Autodesk Inventor part; units mm, degrees
ref_plane "YZ Plane" through (0, 0, 0) normal (1, 0, 0) x (0, 1, 0)
ref_plane "XZ Plane" through (0, 0, 0) normal (0, 1, 0) x (-1, 0, 0)
ref_plane "XY Plane" through (0, 0, 0) normal (0, 0, 1) x (1, 0, 0)
sketch "Sketch1" plane through (0, 0, 0) normal (0, 1, 0) x (-1, 0, 0)
  line L0 (58, 27) -> (-58, 27)
  line L1 (-58, 27) -> (-58, -27)
  line L2 (-58, -27) -> (58, -27)
  line L3 (58, -27) -> (58, 27)
  line L4 (58, 27) -> (-58, -27) construction
  line L5 (-58, 27) -> (58, -27) construction
  point P0 (0, 0)
  dimension "d0" = 116
  dimension "d1" = 54
extrude "Body" add sketch "Sketch1" along normal mid plane 10
sketch "Sketch2" plane through (0, 5, 0) normal (0, 1, 0) x (1, 0, 0)
  line L0 (-55.75, 18.75) -> (55.75, 18.75)
  line L1 (55.75, 18.75) -> (55.75, -18.75)
  line L2 (55.75, -18.75) -> (-55.75, -18.75)
  line L3 (-55.75, -18.75) -> (-55.75, 18.75)
  line L4 (-55.75, 18.75) -> (55.75, -18.75) construction
  line L5 (55.75, 18.75) -> (-55.75, -18.75) construction
  point P0 (0, 0)
  dimension "d4" = 111.5
  dimension "d5" = 37.5
extrude "Top Socket" cut sketch "Sketch2" against normal blind 2
sketch "Sketch3" plane through (0, 3, 0) normal (0, 1, 0) x (1, 0, 0)
  line L0 (-8, -9) -> (8, -9)
  line L1 (8, -9) -> (8, 9)
  line L2 (8, 9) -> (-8, 9)
  line L3 (-8, 9) -> (-8, -9)
  line L4 (-8, -9) -> (8, 9) construction
  line L5 (8, -9) -> (-8, 9) construction
  point P0 (0, 0)
  dimension "d29" = 18
  dimension "d30" = 16
extrude "Photoelectrode Bay" cut sketch "Sketch3" against normal blind 2
sketch "Sketch4" plane through (0, 3, 0) normal (0, 1, 0) x (1, 0, 0)
  circle A0 centre (14, 0) radius 1.45
  line L0 (-55.75, -18.75) -> (-55.75, 18.75)
  line L1 (-55.75, 0) -> (55.75, 0)
  line L2 (55.75, 18.75) -> (55.75, -18.75)
  line L3 (-55.75, -3) -> (55.75, -3)
  line L4 (8, 9) -> (8, -9)
  point P0 (0, 0)
  dimension "d11" = 2.9
  dimension "d20" = 3
  dimension "d97" = 6
revolve "Ref elec" cut sketch "Sketch4" angle 90 about axis through (-55.75, 3, 3) along (-1, 0, 0) contours L1 A0 | A0 L1
sketch "Sketch7" plane through (-58, 5, 27) normal (0, 0, 1) x (1, 0, 0)
  circle A0 centre (72, -5) radius 1.45
  circle A1 centre (72, -5) radius 1.45
  point P0 (58, -5)
  dimension "d21" = 2.9
extrude "Ref elec length" cut sketch "Sketch7" against normal up to surface (24 mm away)
sketch "Sketch8" plane through (-58, 5, 27) normal (0, 0, 1) x (1, 0, 0)
  line L0 (116, -10) -> (0, -10)
  line L1 (113.75, 0) -> (2.25, 0)
  line L2 (64.5, 0) -> (79.5, 0)
  line L3 (79.5, 0) -> (79.5, -10)
  line L4 (79.5, -10) -> (64.5, -10)
  line L5 (64.5, -10) -> (64.5, 0)
  line L6 (79.5, 0) -> (64.5, -10) construction
  line L7 (116, -10) -> (116, 0)
  point P0 (58, -5)
  point P1 (72, -5)
  point P2 (72, -10)
  dimension "d108" = 15
  dimension "d109" = 0
sketch "Sketch9" plane through (0, 1, 0) normal (0, 1, 0) x (1, 0, 0)
  line L0 (8, -9) -> (-8, -9)
  line L1 (8, -9) -> (-8, -9)
  line L2 (-8, -9) -> (8, -9)
  line L3 (8, -9) -> (8, -5.5)
  line L4 (8, -5.5) -> (-8, -5.5)
  line L5 (-8, -5.5) -> (-8, -9)
  dimension "d70" = 3.5
extrude "Photoelectrode Hole" cut sketch "Sketch9" against normal through all
sketch "Sketch12" plane through (0, 5, 0) normal (0, 1, 0) x (1, 0, 0)
  line L0 (58, 27) -> (-58, 27)
  circle A0 centre (-50.8, 25.4) radius 6
  line L1 (-58, -27) -> (-58, 27)
  line L2 (-58, 0) -> (58, 0)
  line L3 (58, 27) -> (58, -27)
  line L4 (-58, -27) -> (58, -27)
  line L5 (0, -27) -> (0, 27)
  circle A1 centre (50.8, 25.4) radius 6
  circle A2 centre (-50.8, -25.4) radius 6
  circle A3 centre (50.8, -25.4) radius 6
  line L6 (-50.8, 25.4) -> (50.8, 25.4)
  line L7 (-50.8, -25.4) -> (50.8, -25.4)
  circle A4 centre (0, 25.4) radius 6
  circle A5 centre (0, -25.4) radius 6
  point P0 (0, 0)
  dimension "d40" = 25.4
  dimension "d49" = 50.8
  dimension "d57" = 12
extrude "Screw clamp boss" add sketch "Sketch12" against normal up to surface (10 mm away) contours A1 L0 | L0 A1 | A4 L6 L5 L0 | L0 A4 | A5 L7 L5 | L5 L7 A5 | A4 L6 L5 | L5 L6 A4 | A3 L4 | L4 A3 | L5 L6 A4 L0 | L7 A5 L4 L5 | L5 L4 A5 L7 | A0 L0 | L0 A0 | A2 L4 | L4 A2 | L4 A5
sketch "Sketch15" plane through (0, 5, 0) normal (0, 1, 0) x (1, 0, 0)
  circle A0 centre (0, 25.4) radius 3.5
  arc A1 (5.7827, 27) -> (-5.7827, 27) centre (0, 25.4) ccw
  circle A2 centre (-50.8, 25.4) radius 3.5
  arc A3 (-45.0173, 27) -> (-56.5827, 27) centre (-50.8, 25.4) ccw
  line L0 (55.75, -18.75) -> (-55.75, -18.75)
  line L1 (0, -18.75) -> (0, 18.75)
  line L2 (-55.75, 18.75) -> (55.75, 18.75)
  line L3 (-58, 27) -> (-58, -27)
  line L4 (-58, 0) -> (58, 0)
  line L5 (58, -27) -> (58, 27)
  circle A4 centre (50.8, 25.4) radius 3.5
  circle A5 centre (0, -25.4) radius 3.5
  circle A6 centre (-50.8, -25.4) radius 3.5
  circle A7 centre (50.8, -25.4) radius 3.5
  point P0 (0, 0)
  dimension "d60" = 7
extrude "Screw Clamp Hole" cut sketch "Sketch15" against normal through all
sketch "Sketch18" plane through (-0.0162, 3, 0) normal (0, 1, 0) x (1, 0, 0)
  line L0 (-45, -15) -> (45, -15)
  line L1 (50, -10) -> (50, 10)
  line L2 (45, 15) -> (-45, 15)
  line L3 (-50, 10) -> (-50, -10)
  line L4 (-50, -15) -> (50, 15) construction
  line L5 (50, -15) -> (-50, 15) construction
  line L6 (-45, -15.5) -> (45, -15.5)
  line L7 (50.5, -10) -> (50.5, 10)
  line L8 (45, 15.5) -> (-45, 15.5)
  line L9 (-50.5, 10) -> (-50.5, -10)
  line L10 (-50.5, -15.5) -> (50.5, 15.5) construction
  line L11 (50.5, -15.5) -> (-50.5, 15.5) construction
  arc A0 (-50, -10) -> (-45, -15) centre (-45, -10) ccw
  arc A1 (45, -15) -> (50, -10) centre (45, -10) ccw
  arc A2 (50, 10) -> (45, 15) centre (45, 10) ccw
  arc A3 (-45, 15) -> (-50, 10) centre (-45, 10) ccw
  arc A4 (-50.5, -10) -> (-45, -15.5) centre (-45, -10) ccw
  arc A5 (45, -15.5) -> (50.5, -10) centre (45, -10) ccw
  arc A6 (50.5, 10) -> (45, 15.5) centre (45, 10) ccw
  arc A7 (-45, 15.5) -> (-50.5, 10) centre (-45, 10) ccw
  point P0 (0, 0)
  dimension "d83" = 100
  dimension "d84" = 30
  dimension "d85" = 0.5
  dimension "d86" = 0.5
  dimension "d87" = 5
  dimension "d88" = 5
  dimension "d89" = 5
  dimension "d90" = 5
  dimension "d91" = 5.5
  dimension "d92" = 5.5
  dimension "d93" = 5.5
  dimension "d94" = 5.5
extrude "Knife Edge" add sketch "Sketch18" along normal blind 1
extrude "Ref Electrode Outlet" add sketch "Sketch8" along normal blind 15
sketch "Sketch19" plane through (45.0173, -5, 27) normal (0, 0, 1) x (1, 0, 0)
  circle A0 centre (-31.0173, 5) radius 1.45
  circle A1 centre (-31.0173, 5) radius 1.45
  line L0 (0, 10) -> (-39.2345, 10)
  line L1 (-29.5673, 10) -> (-18.6963, 10)
  line L2 (-23.5173, 10) -> (0, 10)
  point P0 (-45.0173, 5)
extrude "Extrusion22" cut sketch "Sketch19" along normal blind 9.5
sketch "Sketch20" plane through (0, 5, 0) normal (0, 1, 0) x (1, 0, 0)
  circle A0 centre (14, -35.05) radius 1.45
  circle A1 centre (14, 0) radius 1.45
  line L0 (12.55, -36.5) -> (15.45, -36.5)
  point P0 (0, 0)
extrude "Extrusion23" cut sketch "Sketch20" against normal blind 5 contours A0
sketch "Sketch21" plane through (0, 5, 0) normal (0, 1, 0) x (1, 0, 0)
  circle A0 centre (14, -35.05) radius 4
  circle A1 centre (14, -35.05) radius 1.45
  line L0 (10, -39.05) -> (18, -39.05)
  line L1 (18, -39.05) -> (18, -31.05)
  line L2 (18, -31.05) -> (10, -31.05)
  line L3 (10, -31.05) -> (10, -39.05)
  line L4 (10, -39.05) -> (18, -31.05) construction
  line L5 (18, -39.05) -> (10, -31.05) construction
  point P0 (0, 0)
  dimension "d105" = 8
extrude "Extrusion24" add sketch "Sketch21" along normal blind 5
properties part number "Bottom 6_12"
Could you check a few things on this model? Use its own coordinates, in mm. A direction names the side the tool comes from. Coordinates: 2 decimals unless noted, no trailing zeros. Write each loop counter-clockwise with the first axis right and the second up, starting at its lowest first coordinate (ties: lowest second). Pieces come first, ordered by that corner, then holes. Notation, with made-up numbers: (37.5, 34) - (79.5, 34) arc R23 cw to (79.5, 58) - close; hole circle Ø10 at (-28.5, -26.75). An arc over 180 degrees is marked (long way). Use a Markdown table: item, result.
Q1. I'm going to push flat-ended pins straight in: pin 1 Ø10 at (x, z) = (19.5, -15) entering from +Y; pin 2 Ø4 at (x, y) = (-39.5, 7.5) entering from -Z; pin 3 Ø0.6 at (x, y) = (-2, 1.5) entering from +Z; pin 4 Ø2.5 at (x, y) = (14, 0) entering from -Z. Where does each tip first touch, or does it pass through?
Geometry check:
| item | result |
|---|---|
| pin 1 | stops at y = 5 |
| pin 2 | passes through |
| pin 3 | stops at z = 31.15 |
| pin 4 | stops at z = -27 |
Q2. Imagine slicing it at C-C (x = -31). List the corners of the cut face in (y, z) for me.
Geometry check:
| item | result |
|---|---|
| outline | (-5, -27) - (5, -27) - (5, -18.75) - (3, -18.75) - (3, -15.5) - (4, -15.5) - (4, -15) - (3, -15) - (3, 15) - (4, 15) - (4, 15.5) - (3, 15.5) - (3, 18.75) - (5, 18.75) - (5, 27) - (-5, 27) - close |
Q3. Please list where these lines run through material, in increasing order: L1, parallel to Z at x = 0, y = 0.5; L2, parallel to X at y = -2.25, z = -25.4; L3, parallel to X at y = 0, z = 10.5.
Geometry check:
| item | result |
|---|---|
| L1 | z = -31.4 to -28.9, -21.9 to 5.5, 9 to 21.9, 28.9 to 31.4 |
| L2 | x = -58 to -54.3, -47.3 to -3.5, 3.5 to 47.3, 54.3 to 58 |
| L3 | x = -58 to 12.55, 15.45 to 58 |
Q4. Thinking about a two-plate mould opening in X: for faces 1 (the cylindrical face through (-0.1, 0.1, 31.4)), 2 (the flat face through (18, 7, 35)), 3 (the flat face through (-58, 0, 0)), 4 (the flat face through (1, -5, 5)), which applies, +X half, -X half, draft (parallel to the pull), parting line (faces both ways), or undercut?
Geometry check:
| item | result |
|---|---|
| face 1 | undercut |
| face 2 | +X half |
| face 3 | -X half |
| face 4 | draft |
Q5. Imagine slicing it at A-A (x = 0). Count the separate pieces of the cut face and the enclosed holes in it, and give its area (3 significant figures).
Geometry check:
| item | result |
|---|---|
| separate pieces | 4 |
| enclosed holes | 0 |
| area | 357 mm2 |
Q6. Which directions (+Z, -Z, +X, -X, +Y, -Y) give clear straight access to the entire face, cutting with the end or side of a thin tool? Please do faces 5 (the flat face through (14, 7, 31.05)), 6 (the flat face through (-25, 0, -27)), 7 (the flat face through (-26, 0, 27)), 8 (the flat face through (0, 3, -17)).
Geometry check:
| item | result |
|---|---|
| face 5 | -Z, +X, -X, +Y |
| face 6 | -Z, +Y, -Y |
| face 7 | +Z, +Y, -Y |
| face 8 | +Y |
Q7. Imagine slicing it at B-B (y = 8). List the corners of the cut face in (x, z) for me.
Geometry check:
| item | result |
|---|---|
| outline | (10, 31.05) - (18, 31.05) - (18, 39.05) - (10, 39.05) - close; hole circle Ø2.9 at (14, 35.05) |
